Check sheet for the drawn part. Datum: minimum x, y, z corner. Units: mm. Round coordinates to 2 decimals unless told otherwise and drop trailing zeros. Write each loop counter-clockwise with the first axis right and the second up, starting at its lowest first coordinate (ties: lowest second). Pieces come first, ordered by that corner, then holes. Notation, with made-up numbers: M 38.5,35 L 61.5,35 A13 ccw 61.5,60 Z; hole C 86.25,18.25 d9. An arc over 180 degrees is marked long. One line per item, written item: value.
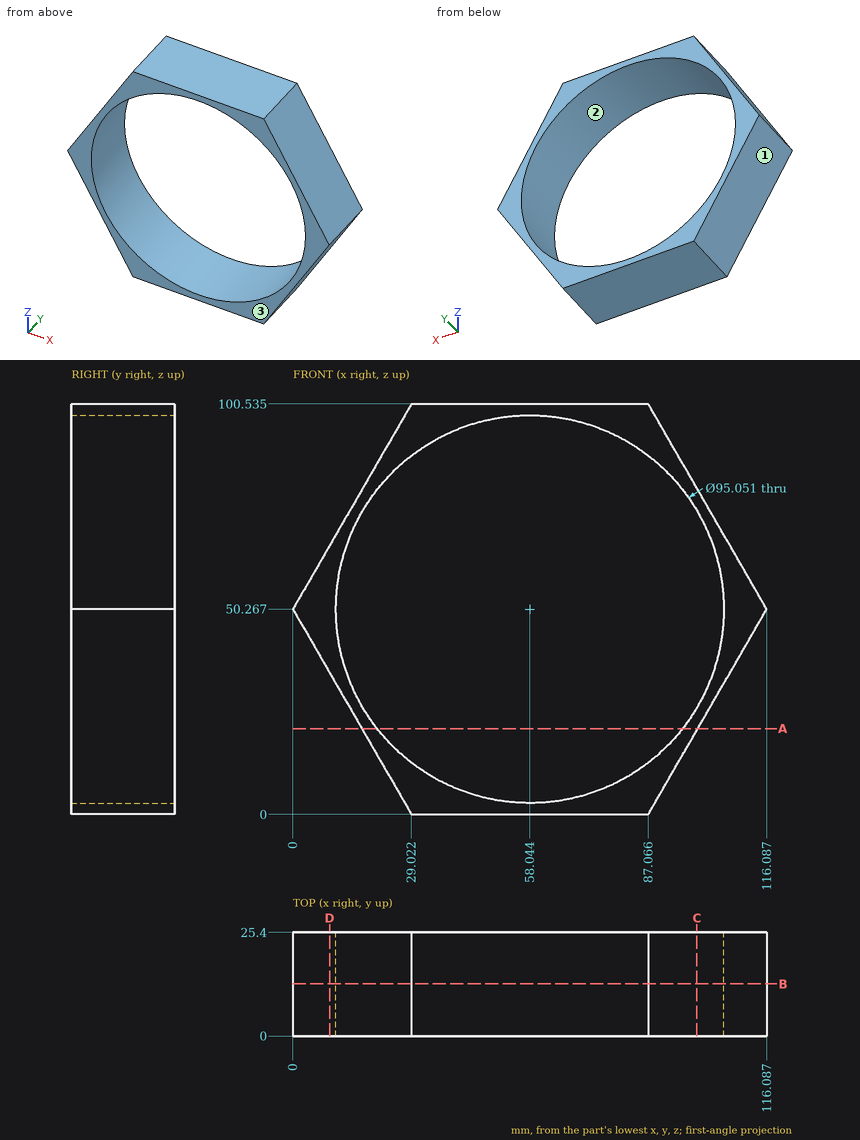
Q1. Sectioned sample at D-D on x = 9. Enter the section's corners in (y, z) (1 decimal), and give its area (3 significant figures).
Completed:
outline: M 0,34.7 L 25.4,34.7 L 25.4,65.9 L 0,65.9 Z
area: 792 mm^2
Q2. Draft check along X on the marked faces 1, 2 and 3. Enter one of: pulls with the +X half, pulls with the -X half, needs draft (parallel to the pull), parting line crosses it, or undercut.
Completed:
face 1: pulls with the -X half
face 2: undercut
face 3: needs draft
Q3. Sectioned sample at B-B on y = 12.75. Enter the section's corners in (x, z) (1 decimal), and give its area (3 significant figures).
Completed:
outline: M 0,50.3 L 29,0 L 87.1,0 L 116.1,50.3 L 87.1,100.5 L 29,100.5 Z; hole C 58,50.3 d95.1
area: 1,660 mm^2
Q4. Sectioned sample at A-A on z = 21. Enter the section's corners in (x, y), and give its area (3 significant figures).
Completed:
outline: M 16.9,0 L 20.6,0 L 20.6,25.4 L 16.9,25.4 Z; M 95.49,0 L 99.19,0 L 99.19,25.4 L 95.49,25.4 Z
area: 188 mm^2
Q5. Scan lines: line 1 (Z direction, x = 59.5, y = 19) (1 decimal); line 2 (Z direction, x = 67.5, y = 8) (1 decimal); line 3 (X direction, y = 23.5, z = 60.5) (1 decimal). Record each from-to range of solid material in increasing order. Write a range as [from, to].
Completed:
line 1: [0, 2.8], [97.8, 100.5]
line 2: [0, 3.7], [96.8, 100.5]
line 3: [5.9, 11.6], [104.5, 110.2]
Q6. Sectioned sample at C-C on x = 99. Enter the section's corners in (y, z), and give its area (3 significant figures).
Completed:
outline: M 0,20.67 L 25.4,20.67 L 25.4,26.16 L 0,26.16 Z; M 0,74.38 L 25.4,74.38 L 25.4,79.86 L 0,79.86 Z
area: 279 mm^2
Q7. Depth check by flat-ended pin: P1, Ø5, axis at x = 33, y = 12.5, coming from the -Z side; P2, Ø8, axis at y = 20, z = 29.5, coming from the -X side; P3, Ø5, axis at y = 5.5, z = 56, coming from the +X side; P4, Ø4, axis at y = 12.5, z = 14, coming from the +X side. Enter the tip coordinate at first touch or a pass-through.
Completed:
P1: z = 0
P2: x = 9.68
P3: x = 114.22
P4: x = 96.3
